Design review of the part built by this model. Coordinates are the model's own, in mm. A direction names the side the tool comes from. Round coordinates to 2 decimals unless told otherwise and drop trailing zeros. Write each loop counter-clockwise with the first axis right and the second up, starting at its lowest first coordinate (ties: lowest second). Pieces come first, ordered by that corner, then holes. Notation, with made-up numbers: (-9, 68) -> (26, 68) arc R21 ccw to (26, 106) -> close; hole circle Ø6 at (85, 81). An arc over 180 degrees is marked (long way). Write item = value, one per line. Start each with the question number.
Item 1: To check wall thickness, follow L1, parallel to Z at x = -10.5, y = -11; L2, parallel to Z at x = -4, y = 6; L3, parallel to Y at x = -6, z = 103. State the ranges of each line that lie inside material, in increasing order.
Item 2: Add section A-A, the plane x = 0. State the section outline as (y, z) points.
Item 3: Machinability: for faces 1 (the cylindrical face through (-4.336, -19.524, 12.353)), 2 (the cylindrical face through (-7.493, 0.33, 128.065)), which of the approach directions +Z, -Z, +X, -X, +Y, -Y give a long, thin tool a straight path to every point of the face, cutting with its end or side? Answer none if there is none.
Item 4: For pin 1 Ø8 at (y, z) = (3, 157.5) entering from -X; pin 2 Ø1 at (y, z) = (-2, 114.5) entering from -X; pin 3 Ø1.5 at (x, y) = (-2, -9) entering from +Z; pin 4 Ø8 at (x, z) = (15, 194) entering from +Y, all flat-tipped, find the tip position at first contact; note any pin that passes through.
Item 5: Add section C-C, the plane z = 177.5. State the section outline as (x, y) points.
from build123d import *

# Parameters (mm, degrees)
F0_R     = 20
F1_DEPTH = 25
F2_R     = 7.5
F3_DEPTH = 208
F4_R     = 2
F5_R     = 1


with BuildPart() as f1:
    # F0 (on Top) → F1 (new body)
    with BuildSketch(Plane.XY):
        Circle(F0_R)
    extrude(amount=F1_DEPTH)

    # F2 (on face) → F3 (join)
    with BuildSketch(Plane.XY.offset(25)):
        Circle(F2_R)
    extrude(amount=F3_DEPTH)

    # F4
    f4_edges = [f1.edges().sort_by_distance(p)[0] for p in [
        (-20, 0, 0),
        (-20, 0, 25),
        (-7.5, 0, 25),
    ]]
    fillet(f4_edges, radius=F4_R)

    # F5
    f5_edges = [f1.edges().sort_by_distance(p)[0] for p in [
        (-7.5, 0, 233),
    ]]
    fillet(f5_edges, radius=F5_R)


solid = f1.part
Result set:
q1.L1 = 0 to 25
q1.L2 = 0 to 232.7
q1.L3 = -4.5 to 4.5
q2.outline = (-20, 2) arc R2 ccw to (-18, 0) -> (18, 0) arc R2 ccw to (20, 2) -> (20, 23) arc R2 ccw to (18, 25) -> (9.5, 25) arc R2 cw to (7.5, 27) -> (7.5, 232) arc R1 ccw to (6.5, 233) -> (-6.5, 233) arc R1 ccw to (-7.5, 232) -> (-7.5, 27) arc R2 cw to (-9.5, 25) -> (-18, 25) arc R2 ccw to (-20, 23) -> close
q3.face_1 = +Z, -Z
q3.face_2 = +Z
q4.pin_1 = -7.5
q4.pin_2 = -7.35
q4.pin_3 = 25.29
q4.pin_4 = through
q5.outline = circle Ø15 at (0, 0)
